Check sheet for the modelled part. Datum: model origin and axes. Units: mm. A direction names the side the tool comes from. Round coordinates to 2 decimals unless told otherwise and drop trailing zeros. Write each loop counter-clockwise with the first axis right and the second up, starting at its lowest first coordinate (ties: lowest second). Pieces come first, ordered by that corner, then holes. Notation, with made-up numbers: (78.25, -3.5) -> (124.25, -3.5) arc R29 ccw to (124.25, 19.5) -> close; hole circle Ø7 at (-20, -1). An arc over 180 degrees is marked (long way). One line per item, written item: value.
Autodesk Inventor part; units mm, degrees
ref_plane "YZ Plane" through (0, 0, 0) normal (1, 0, 0) x (0, 1, 0)
ref_plane "XZ Plane" through (0, 0, 0) normal (0, 1, 0) x (-1, 0, 0)
ref_plane "XY Plane" through (0, 0, 0) normal (0, 0, 1) x (1, 0, 0)
sketch "Sketch1" plane through (0, 0, 0) normal (0, 0, 1) x (1, 0, 0)
  line L0 (0, 0) -> (0, 10)
  line L1 (0, 10) -> (6, 10)
  line L2 (6, 10) -> (6, 12.5)
  line L3 (6, 12.5) -> (54, 12.5)
  line L4 (54, 12.5) -> (54, 10)
  line L5 (54, 10) -> (60, 10)
  line L6 (60, 10) -> (60, 0)
  line L7 (60, 0) -> (0, 0)
  dimension "d0" = 10
  dimension "d1" = 6
  dimension "d2" = 2.5
  dimension "d3" = 48
  dimension "d4" = 2.5
  dimension "d5" = 6
  dimension "d6" = 10
revolve "Revolution1" add sketch "Sketch1" angle 360 about axis through (60, 0, 0) along (-1, 0, 0)
sketch "Sketch2" plane through (60, 0, 0) normal (1, 0, 0) x (0, 0, -1)
  point P0 (0, 0)
  point P1 (-32.9803, -18.1231)
properties part number "roller pin"
Item 1: Release check for a two-part mould opening along Y. For faces 4 (the cylindrical face through (57.04, -2.17, -9.76)), 5 (the flat face through (6, -0.1, -10.2)) record: pulls with the +Y half, pulls with the -Y half, needs draft (parallel to the pull), parting line crosses it, or undercut.
Result set:
face 4: parting line crosses it
face 5: needs draft
Item 2: Tool access check on faces 1 (the cylindrical face through (30.336, 11.923, 3.755)), 2 (the flat face through (54, -0.1, -10.2)), 3 (the cylindrical face through (3.04, -2.17, -9.76)). Record the directions out of +Z, -Z, +X, -X, +Y, -Y that give a thin tool (end or side, any length) a straight path to the whole face; none if there is none.
Result set:
face 1: +X, -X
face 2: +X
face 3: -X
Item 3: Depth check by flat-ended pin: pin 1 (4 mm diameter, centred on y = 0.5, z = 0, fed in from -X); pin 2 (5 mm diameter, centred on x = 47, y = 6.5, fed in from +Z); pin 3 (3 mm diameter, centred on x = 40.5, y = 3, fed in from +Z); pin 4 (2 mm diameter, centred on x = 47.5, y = -9, fed in from +Z). Enter the tip coordinate at first touch or a pass-through.
Result set:
pin 1: x = 0
pin 2: z = 11.84
pin 3: z = 12.41
pin 4: z = 9.6
Item 4: Material ranges on line 1 along X through (y, z) = (10, -1.5); line 2 along Z through (x, y) = (27, -0.25); line 3 along Z through (x, y) = (4, 0.5), recorded low to high.
Result set:
line 1: 6 to 54
line 2: -12.5 to 12.5
line 3: -9.99 to 9.99
Item 5: Sectioned sample at D-D (x = 14.5). Enter the section's corners in (y, z).
Result set:
outline: circle Ø25 at (0, 0)
Item 6: Sectioned sample at C-C (x = 56). Enter the section's corners in (y, z), then the cut area to 3 significant figures.
Result set:
outline: circle Ø20 at (0, 0)
area: 314 mm^2
Item 7: Sectioned sample at A-A (z = 0). Enter the section's corners in (x, y), then the cut area to 3 significant figures.
Result set:
outline: (0, -10) -> (6, -10) -> (6, -12.5) -> (54, -12.5) -> (54, -10) -> (60, -10) -> (60, 10) -> (54, 10) -> (54, 12.5) -> (6, 12.5) -> (6, 10) -> (0, 10) -> close
area: 1,440 mm^2
